from build123d import *

# Parameters (mm, degrees)
F1_DEPTH      = 40.132
F2_R          = 13.093188
F3_DEPTH      = 3.048
F3_DEPTH_BACK = 3.556
F7_W          = 33.782
F7_H          = 37.713479
F8_DEPTH      = 8.636


with BuildPart() as f1:
    # F0 (on Right) → F1 (new body)
    with BuildSketch(Plane.YZ):
        Polygon((-79.37751, 10.118734), (-54.077905, 10.751224), (24.140039, 10.751224), (24.140039, 20.027746), (-4.532847, 22.768537), (-10.857747, 38.58079), (-35.314031, 38.58079), (-35.314031, 22.557706), (-79.37751, 22.557706), align=None)
    extrude(amount=F1_DEPTH)

    # F2 (on face) → F3 (join, two sides)
    with BuildSketch(Plane.YZ.offset(40.132)) as f3_sk:
        with Locations((-59.244439, 4.847982)):
            Circle(F2_R)
        with Locations((-4.532847, 4.847982)):
            Circle(F2_R)
    extrude(amount=F3_DEPTH)
    extrude(f3_sk.sketch, amount=-F3_DEPTH_BACK)

    # F6: F1 across plane


with BuildPart() as f1_1:
    add(f1.part)
    add(f1.part.mirror(Plane(origin=(20.066, -10.857747, 38.58079), x_dir=(0, 1, 0), z_dir=(1, 0, 0))))

    # F7 (on face) → F8 (cut)
    with BuildSketch(Plane.XY.offset(22.557706)):
        with Locations((20.066, -57.34577)):
            Rectangle(F7_W, F7_H)
    extrude(amount=-F8_DEPTH, mode=Mode.SUBTRACT)


solid = f1_1.part
Model file for the job. Use its own axes, mm. A direction names the side the tool comes from. Give positions to 0.01 mm unless a question says otherwise; leave off trailing zeros. Order: outer loops, then holes, each group sorted by start corner. A loop starts at its lowest first (then second) coordinate and runs counter-clockwise, first axis right, second up. Notation, with made-up numbers: (49, 88) - (67, 88) arc R20 cw to (67, 117) - close; hole circle Ø6 at (-12, -30.75). An arc over 180 degrees is marked (long way). One line per item, written item: value.
Item 1: Two-plate mould, pull along X, no slides. Class faces 4 (the flat face through (43.18, -5, 5)), 5 (the flat face through (3.175, -58, 18)), 6 (the flat face through (20, -57, 13.922)), 7 (the flat face through (20, -79.378, 16)): released by +X, released by -X, zero draft, split by the parting line, or undercut.
Response values:
face 4: released by +X
face 5: undercut
face 6: undercut
face 7: zero draft
Item 2: Tool access for faces 1 (the flat face through (20, -76.203, 18)), 2 (the flat face through (20, -35.314, 31)), 3 (the cylindrical face through (0.208, -7.371, -7.934)): list every direction of +Z, -Z, +X, -X, +Y, -Y with a clear straight run to the whole face (end or side of a thin tool).
Response values:
face 1: +Z
face 2: +Z, +X, -X, -Y
face 3: -X
Item 3: Wall check: line 1 (X direction, y = -56, z = 21.5) (3 decimals); line 2 (X direction, y = -65, z = 5); line 3 (Y direction, x = 28, z = 18.5). Give the ranges that are in metal, low to high.
Response values:
line 1: 0 to 3.175, 36.957 to 40.132
line 2: -3.05 to 3.56, 36.58 to 43.18
line 3: -79.38 to -76.2, -38.49 to 24.14
Item 4: Slice it at B-B (z = 3.5). List the corners of the cut face in (x, y), then the cut area to 3 significant figures.
Response values:
outline: (-3.05, -72.27) - (3.56, -72.27) - (3.56, -46.22) - (-3.05, -46.22) - close; (-3.05, -17.56) - (3.56, -17.56) - (3.56, 8.49) - (-3.05, 8.49) - close; (36.58, -72.27) - (43.18, -72.27) - (43.18, -46.22) - (36.58, -46.22) - close; (36.58, -17.56) - (43.18, -17.56) - (43.18, 8.49) - (36.58, 8.49) - close
area: 688 mm2
Item 5: Slice it at D-D (z = 16.5). List the corners of the cut face in (x, y) (1 decimal).
Response values:
outline: (-3, -65.2) - (0, -65.2) - (0, -79.4) - (40.1, -79.4) - (40.1, -65.2) - (43.2, -65.2) - (43.2, -53.3) - (40.1, -53.3) - (40.1, -10.5) - (43.2, -10.5) - (43.2, 1.4) - (40.1, 1.4) - (40.1, 24.1) - (0, 24.1) - (0, 1.4) - (-3, 1.4) - (-3, -10.5) - (0, -10.5) - (0, -53.3) - (-3, -53.3) - close; hole (3.2, -76.2) - (37, -76.2) - (37, -38.5) - (3.2, -38.5) - close
Item 6: Slice it at C-C (y = -40). List the corners of the cut face in (x, z) (3 decimals).
Response values:
outline: (0, 10.751) - (40.132, 10.751) - (40.132, 22.558) - (36.957, 22.558) - (36.957, 13.922) - (3.175, 13.922) - (3.175, 22.558) - (0, 22.558) - close
Item 7: Pin check, flat tips, straight feed: pin 1 Ø12 at (x, y) = (18, -68) entering from +Z; pin 2 Ø4 at (x, y) = (4.5, 13.5) entering from +Z; pin 3 Ø10 at (x, z) = (33.5, -0.5) entering from +Y. Stop position of each tip, or through.
Response values:
pin 1: z = 13.92
pin 2: z = 21.24
pin 3: y = 8.48
Item 8: Slice it at A-A (x = 26.5). List the corners of the cut face in (y, z), then the cut area to 3 significant figures.
Response values:
outline: (-79.38, 10.12) - (-54.08, 10.75) - (24.14, 10.75) - (24.14, 20.03) - (-4.53, 22.77) - (-10.86, 38.58) - (-35.31, 38.58) - (-35.31, 22.56) - (-38.49, 22.56) - (-38.49, 13.92) - (-76.2, 13.92) - (-76.2, 22.56) - (-79.38, 22.56) - close
area: 1,310 mm2
